Autodesk Inventor part; units mm, degrees
ref_plane "YZ Plane" through (0, 0, 0) normal (1, 0, 0) x (0, 1, 0)
ref_plane "XZ Plane" through (0, 0, 0) normal (0, 1, 0) x (-1, 0, 0)
ref_plane "XY Plane" through (0, 0, 0) normal (0, 0, 1) x (1, 0, 0)
sketch "Sketch1" plane through (0, 0, 0) normal (0, 1, 0) x (-1, 0, 0)
  line L0 (13.3302, 27.1778) -> (-12.6698, 27.1778)
  line L1 (-12.6698, 27.1778) -> (-12.6698, -9.8222)
  line L2 (-12.6698, -9.8222) -> (13.3302, -9.8222)
  line L3 (13.3302, -9.8222) -> (13.3302, 27.1778)
  line L4 (6.5302, 7.1778) -> (-5.8698, 7.1778)
  line L5 (-5.8698, 7.1778) -> (-5.8698, -9.8222)
  line L6 (-5.8698, -9.8222) -> (6.5302, -9.8222)
  line L7 (6.5302, -9.8222) -> (6.5302, 7.1778)
  line L8 (-12.6698, 27.1778) -> (-8.6698, 27.1778)
  line L9 (-8.6698, 27.1778) -> (-8.6698, -9.8222)
  line L10 (-8.6698, -9.8222) -> (-12.6698, -9.8222)
  line L11 (-12.6698, -9.8222) -> (-12.6698, 27.1778)
  point P0 (0, 0)
  dimension "d0" = 26
  dimension "d1" = 37
  dimension "d2" = 6.8
  dimension "d3" = 6.8
  dimension "d4" = 17
  dimension "d5" = 4
extrude "Extrusion1" add sketch "Sketch1" along normal blind 3 contours L3 L2 L7 L4 L5 L9 L0 | L9 L2 L1 L0
extrude "Extrusion2" add sketch "Sketch1" along normal blind 9 contours L9 L2 L1 L0
sketch "Sketch2" plane through (12.6698, 0, 27.1778) normal (1, 0, 0) x (0, 0, -1)
  circle A0 centre (4, 5) radius 1.9
  circle A1 centre (33, 5) radius 1.9
  line L0 (0, 0) -> (0, 9)
  line L1 (37, 0) -> (37, 9)
  line L2 (0, 0) -> (37, 0)
  point P0 (27.1778, 0)
  dimension "d10" = 3.8
  dimension "d11" = 3.8
  dimension "d12" = 4
  dimension "d13" = 4
  dimension "d14" = 4
  dimension "d15" = 4
  dimension "d27" = 5
  dimension "d28" = 29
extrude "Extrusion3" cut sketch "Sketch2" against normal blind 8
fillet "Fillet1" radius 3 1 edges at (8.6698, 3, 8.6778)
sketch "Sketch3" plane through (-13.3302, 0, 27.1778) normal (0, 0, 1) x (1, 0, 0)
  line L0 (26, 0) -> (13.75, 0.65)
  line L1 (12.25, 0.65) -> (0, 0)
  line L2 (0, 0) -> (26, 0)
  line L3 (0, 0) -> (26, 0)
  line L4 (0, 0) -> (0, 3)
  line L5 (26, 0) -> (26, 9)
  line L6 (13.75, 0.65) -> (12.25, 0.65)
  point P0 (13.3302, 0)
  dimension "d21" = 26
  dimension "d24" = 0.65
  dimension "d25" = 1.5
  dimension "d26" = 12.25
extrude "Extrusion4" cut sketch "Sketch3" against normal blind 40
equation "\"d26\" = 0.5 * d21 - 0.5 * d25"
properties part number "psu rear brace"
The listing builds one solid part. Answer for the finished solid, in the listing's coordinates (mm). A direction names the side the tool comes from. Coordinates: 2 decimals unless noted, no trailing zeros. Loops run counter-clockwise (first coordinate to the right, second up) from the corner with the lowest first, then second, coordinate; pieces in that order, holes last. Notation, with made-up numbers: (-17, 3) -> (-8, 3) arc R29 ccw to (-8, 40) -> close; hole circle Ø2 at (-0.75, 71). An arc over 180 degrees is marked (long way). Answer in a Markdown table with one row per item. Add a question column.
1. Flat-ended cylindrical pins translate along their axes: P1, Ø1.6, axis at x = 0, z = 19, coming from the -Y side; P2, Ø1, axis at y = 7, z = 11, coming from the -X side; P3, Ø0.8, axis at x = 2, y = 2, coming from the -Z side. Find the tip coordinate at first contact, or state that the pin passes through.
2. Determine the mould class of faces 5 (the cylindrical face through (10.289, 3.145, 23.59)), 6 (the flat face through (-6, 3, 13)), 7 (the flat face through (-13.33, 1, 8)) for opening direction Y: +Y half, -Y half, draft (parallel to the pull), parting line (faces both ways), or undercut.
3. The part is cut by section B-B, the plane y = 2.5. Write down the section's boundary in (x, z).
4. The part is cut by section A-A, the plane z = 1.5. Write down the section's boundary in (x, y).
5. The part is cut by section D-D, the plane z = 9.5. Write down the section's boundary in (x, y).
6. Consider line 1 (Z direction, x = 11.25, y = 5); line 2 (X direction, y = 2.5, z = -0.5); line 3 (X direction, y = 8, z = 6). Determine where each line is inside the solid, lowest interval first. Write a range as [from, to].
7. The part is cut by section C-C, the plane x = 9.5. Write down the section's boundary in (y, z).
8. For faces 1 (the flat face through (8.67, 7, 9)), 2 (the cylindrical face through (10.289, 3.145, -5.41)), 3 (the flat face through (-6.53, 2, -1)), 4 (the flat face through (0, 0.65, 17)), determine the directions among +Z, -Z, +X, -X, +Y, -Y from which every point of the face is accessible in a straight line to the end or side of a thin tool.
Answer below:
| question | item | result |
|---|---|---|
| 1 | P1 | y = 0.63 |
| 1 | P2 | x = 8.67 |
| 1 | P3 | z = 7.18 |
| 2 | face 5 | undercut |
| 2 | face 6 | +Y half |
| 2 | face 7 | draft |
| 3 | outline | (-13.33, -9.82) -> (-6.53, -9.82) -> (-6.53, 7.18) -> (5.87, 7.18) -> (5.87, -9.82) -> (12.67, -9.82) -> (12.67, 27.18) -> (-13.33, 27.18) -> close |
| 4 | outline | (-13.33, 0) -> (-6.53, 0.36) -> (-6.53, 3) -> (-13.33, 3) -> close; (5.87, 0.36) -> (12.67, 0) -> (12.67, 9) -> (8.67, 9) -> (8.67, 6) arc R3 cw to (5.87, 3.01) -> close |
| 5 | outline | (-13.33, 0) -> (-1.08, 0.65) -> (0.42, 0.65) -> (12.67, 0) -> (12.67, 9) -> (8.67, 9) -> (8.67, 6) arc R3 cw to (5.67, 3) -> (-13.33, 3) -> close |
| 6 | line 1 | [-9.82, -7.72], [-3.92, 21.28], [25.08, 27.18] |
| 6 | line 2 | [-13.33, -6.53], [5.87, 12.67] |
| 6 | line 3 | [8.67, 12.67] |
| 7 | outline | (0.17, -9.82) -> (9, -9.82) -> (9, 27.18) -> (0.17, 27.18) -> close; hole circle Ø3.8 at (5, -5.82); hole circle Ø3.8 at (5, 23.18) |
| 8 | face 1 | +Z, -Z, -X, +Y |
| 8 | face 2 | +X, -X |
| 8 | face 3 | -Z, +Y, -Y |
| 8 | face 4 | +Z, -Z, -Y |
